Autodesk Inventor part; units mm, degrees
ref_plane "YZ Plane" through (0, 0, 0) normal (1, 0, 0) x (0, 1, 0)
ref_plane "XZ Plane" through (0, 0, 0) normal (0, 1, 0) x (-1, 0, 0)
ref_plane "XY Plane" through (0, 0, 0) normal (0, 0, 1) x (1, 0, 0)
sketch "Эскиз1" plane through (0, 0, 0) normal (0, 0, 1) x (1, 0, 0)
  line L0 (-39.5, -20) -> (39.5, -20)
  line L1 (39.5, -20) -> (39.5, 20)
  line L2 (39.5, 20) -> (-39.5, 20)
  line L3 (-39.5, 20) -> (-39.5, -20)
  line L4 (-39.5, -20) -> (39.5, 20) construction
  line L5 (39.5, -20) -> (-39.5, 20) construction
  line L6 (-38.5, 19) -> (38.5, 19)
  line L7 (38.5, 19) -> (38.5, -19)
  line L8 (38.5, -19) -> (-38.5, -19)
  line L9 (-38.5, -19) -> (-38.5, 19)
  point P0 (0, 0)
  dimension "d0" = 79
  dimension "d1" = 40
  dimension "d2" = 1
extrude "Выдавливание1" add sketch "Эскиз1" along normal blind 3 contours L6 L7 L8 L9
extrude "Выдавливание2" add sketch "Эскиз1" along normal blind 20
sketch "Эскиз2" plane through (-39.5, -20, 0) normal (0, -1, 0) x (1, 0, 0)
  line L0 (2, 20) -> (2, 16) construction
  line L1 (4, 14) -> (11, 14)
  arc A0 (2, 16) -> (4, 14) centre (4, 16) ccw
  line L2 (11, 14) -> (11, 9) construction
  line L3 (14.3166, 9) -> (22.3166, 9)
  line L4 (24.3166, 7) -> (24.3166, 4)
  arc A1 (24.3166, 7) -> (22.3166, 9) centre (22.3166, 7) ccw
  line L5 (24.3166, 4) -> (39.5, 4)
  line L6 (39.5, 0) -> (39.5, 20) construction
  line L7 (77, 20) -> (77, 16) construction
  line L8 (75, 14) -> (68, 14)
  arc A2 (75, 14) -> (77, 16) centre (75, 16) ccw
  line L9 (68, 14) -> (64.6834, 9)
  line L10 (64.6834, 9) -> (56.6834, 9)
  line L11 (54.6834, 7) -> (54.6834, 4)
  arc A3 (56.6834, 9) -> (54.6834, 7) centre (56.6834, 7) ccw
  line L12 (54.6834, 4) -> (39.5, 4)
  line L13 (77, 20) -> (77, 16) construction
  line L14 (77, 20) -> (77, 16)
  line L15 (2, 20) -> (77, 20)
  line L16 (14.3166, 9) -> (22.3166, 9)
  line L17 (24.3166, 7) -> (24.3166, 4)
  line L18 (24.3166, 4) -> (54.6834, 4)
  line L19 (54.6834, 4) -> (54.6834, 7)
  line L20 (56.6834, 9) -> (64.6834, 9)
  line L21 (64.6834, 9) -> (68, 14)
  line L22 (68, 14) -> (75, 14)
  line L23 (77, 16) -> (77, 20)
  line L24 (77, 20) -> (2, 20)
  line L25 (11, 14) -> (14.3166, 9)
  line L26 (2, 20) -> (2, 16)
  line L27 (0, 20) -> (79, 20)
  point P0 (24.3166, 9)
  dimension "d10" = 2
  dimension "d11" = 5
  dimension "d12" = 6
  dimension "d13" = 10
  dimension "d14" = 5
  dimension "d15" = 2
extrude "Выдавливание3" cut sketch "Эскиз2" against normal up to surface (40 mm away)
sketch "Эскиз3" plane through (0, 0, 3) normal (0, 0, 1) x (1, 0, 0)
  line L0 (38.5, 19) -> (-38.5, 19)
  line L1 (-38.5, 19) -> (-38.5, -19)
  line L2 (-38.5, -19) -> (38.5, -19)
  line L3 (38.5, -19) -> (38.5, 19)
  line L4 (-39.5, 20) -> (-39.5, -20)
  line L5 (39.5, 0.5) -> (-39.5, 0.5)
  line L6 (-39.5, 0.5) -> (-39.5, -0.5)
  line L7 (-39.5, -0.5) -> (39.5, -0.5)
  line L8 (39.5, -0.5) -> (39.5, 0.5)
  line L9 (39.5, 0.5) -> (-39.5, -0.5) construction
  line L10 (-39.5, 0.5) -> (39.5, -0.5) construction
  point P0 (0, 0)
  dimension "d18" = 1
extrude "Выдавливание4" add sketch "Эскиз3" along normal blind 10 contours L5 L8 L7 L3 | L3 L7 L1 L5 | L1 L7 L4 L5
properties part number "Badrepack"
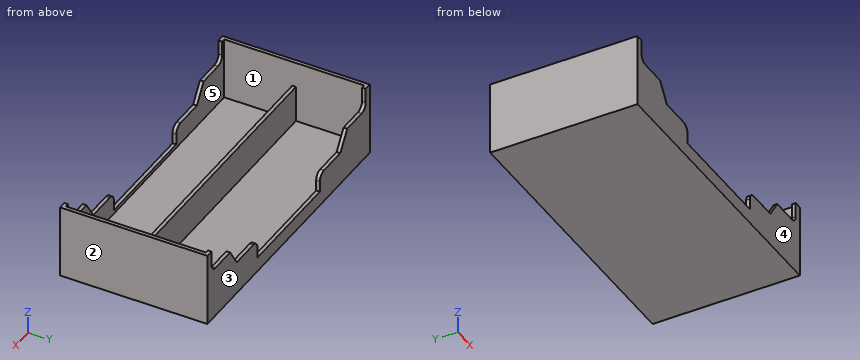
Work out the finished part from the listing and answer in its coordinate system (mm). Face numbers are marked on the shaded views. A direction names the side the tool comes from. Give positions to 0.01 mm unless a question says otherwise; leave off trailing zeros. Loops run counter-clockwise (first coordinate to the right, second up) from the corner with the lowest first, then second, coordinate; pieces in that order, holes last. Notation, with made-up numbers: (48, -11.75) -> (65, -11.75) arc R33 cw to (65, 23.25) -> close; hole circle Ø7 at (26.25, 31). An arc over 180 degrees is marked (long way). Use a Markdown table: item, result. Add a question column.
1. For the marked faces 4 and 5, determine the directions among +Z, -Z, +X, -X, +Y, -Y from which every point of the face is accessible in a straight line to the end or side of a thin tool.
2. Section A-A on z = 17.25 is taken. Determine the outline of the cut face in (x, y).
3. Section C-C on y = -10.5 is taken. Determine the outline of the cut face in (x, z).
4. Section D-D on z = 6 is taken. Determine the outline of the cut face in (x, y).
5. Section B-B on x = 33.5 is taken. Determine the outline of the cut face in (y, z), and give its area (3 significant figures).
6. Determine the mould class of the marked faces 1, 2 and 3 for opening direction X: released by +X, released by -X, zero draft, split by the parting line, or undercut.
7. Flat-ended cylindrical pins translate along their axes: pin 1 Ø2 at (x, z) = (7, 13.5) entering from -Y; pin 2 Ø0.5 at (x, y) = (32, 19.5) entering from +Z; pin 3 Ø1.1 at (x, y) = (-23, -19.5) entering from +Z. Find the tip coordinate at first contact, or state that the pin passes through.
8. Find the intervals of material crossed by probe 1 along Y at (x, z) = (-25, 4.5); probe 2 along X at (y, z) = (5.5, 12.25); probe 3 along Z at (x, y) = (-26, -8), in increasing order.
Results below:
| question | item | result |
|---|---|---|
| 1 | face 4 | +Z, -Z, +X, -X, -Y |
| 1 | face 5 | +Z |
| 2 | outline | (-39.5, -20) -> (-37.5, -20) -> (-37.5, -19) -> (-38.5, -19) -> (-38.5, 19) -> (-37.5, 19) -> (-37.5, 20) -> (-39.5, 20) -> close; (37.5, -20) -> (39.5, -20) -> (39.5, 20) -> (37.5, 20) -> (37.5, 19) -> (38.5, 19) -> (38.5, -19) -> (37.5, -19) -> close |
| 3 | outline | (-39.5, 0) -> (39.5, 0) -> (39.5, 20) -> (38.5, 20) -> (38.5, 3) -> (-38.5, 3) -> (-38.5, 20) -> (-39.5, 20) -> close |
| 4 | outline | (-39.5, -20) -> (-15.18, -20) -> (-15.18, -19) -> (-38.5, -19) -> (-38.5, -0.5) -> (38.5, -0.5) -> (38.5, -19) -> (15.18, -19) -> (15.18, -20) -> (39.5, -20) -> (39.5, 20) -> (15.18, 20) -> (15.18, 19) -> (38.5, 19) -> (38.5, 0.5) -> (-38.5, 0.5) -> (-38.5, 19) -> (-15.18, 19) -> (-15.18, 20) -> (-39.5, 20) -> close |
| 5 | outline | (-20, 0) -> (20, 0) -> (20, 14) -> (19, 14) -> (19, 3) -> (0.5, 3) -> (0.5, 13) -> (-0.5, 13) -> (-0.5, 3) -> (-19, 3) -> (-19, 14) -> (-20, 14) -> close |
| 5 | area | 152 mm^2 |
| 6 | face 1 | undercut |
| 6 | face 2 | released by +X |
| 6 | face 3 | zero draft |
| 7 | pin 1 | stops at y = -0.5 |
| 7 | pin 2 | stops at z = 14 |
| 7 | pin 3 | stops at z = 9 |
| 8 | probe 1 | y = -20 to -19, -0.5 to 0.5, 19 to 20 |
| 8 | probe 2 | x = -39.5 to -38.5, 38.5 to 39.5 |
| 8 | probe 3 | z = 0 to 3 |
